from build123d import *

# Parameters (mm, degrees)
SKETCH_1_R          = 10
EXTRUDE_1_DEPTH     = 65
CUT_EXTRUDE_1_DEPTH = 2.5
SKETCH_3_R          = 17.5
EXTRUDE_2_DEPTH     = 28
SKETCH_4_R          = 1.4
CUT_EXTRUDE_2_DEPTH = 3
SKETCH_5_R          = 1.5
CUT_EXTRUDE_3_DEPTH = 3


with BuildPart() as part:
    # 草图1 → 凸台-拉伸1 (new body)
    with BuildSketch(Plane.XY):
        Circle(SKETCH_1_R)
    extrude(amount=EXTRUDE_1_DEPTH)

    # 草图2 → 切除-拉伸1 (cut)
    with BuildSketch(Plane.ZY.offset(10)):
        with BuildLine():
            Line((30.6, 2.55), (37.6, 2.55))
            ThreePointArc((37.6, 2.55), (40.15, 0), (37.6, -2.55))
            Line((37.6, -2.55), (30.6, -2.55))
            ThreePointArc((30.6, -2.55), (28.05, 0), (30.6, 2.55))
        make_face()
    extrude(amount=-CUT_EXTRUDE_1_DEPTH, mode=Mode.SUBTRACT)

    # 草图3 → 凸台-拉伸2 (add)
    with BuildSketch(Plane(origin=(0, 0, 0), x_dir=(-1, 0, 0), z_dir=(0, 0, -1))):
        Circle(SKETCH_3_R)
    extrude(amount=-EXTRUDE_2_DEPTH)

    # 草图4 → 切除-拉伸2 (cut)
    with BuildSketch(Plane.XY.offset(65)):
        with Locations((0, 7)):
            Circle(SKETCH_4_R)
        with Locations((7, 0)):
            Circle(SKETCH_4_R)
        with Locations((0, -7)):
            Circle(SKETCH_4_R)
        with Locations((-7, 0)):
            Circle(SKETCH_4_R)
    extrude(amount=-CUT_EXTRUDE_2_DEPTH, mode=Mode.SUBTRACT)

    # 草图5 → 切除-拉伸3 (cut)
    with BuildSketch(Plane.XY.offset(65)):
        Circle(SKETCH_5_R)
    extrude(amount=-CUT_EXTRUDE_3_DEPTH, mode=Mode.SUBTRACT)


solid = part.part
Input: part model. Units: mm. Frame: model coordinates. A direction names the side the tool comes from. Coordinates: 2 decimals unless noted, no trailing zeros. Order: outer loops, then holes, each group sorted by start corner. A loop starts at its lowest first (then second) coordinate and runs counter-clockwise, first axis right, second up. Notation, with made-up numbers: M 51,58 L 100,58 A8 cw 100,67 Z; hole C 83.25,35.25 d5. An arc over 180 degrees is marked long. Answer as CSV lines item,"result".
1. Section B-B (x = -3). Return the cut outline in (y, z).
Reported:
outline,"M -17.24,0 L 17.24,0 L 17.24,28 L 9.54,28 L 9.54,65 L -9.54,65 L -9.54,28 L -17.24,28 Z"
2. First-contact query: P1, Ø2.5, axis at x = 7, y = 0, coming from the +Z side; P2, Ø1.7, axis at x = -9, z = 35, coming from the -Y side; P3, Ø2, axis at y = 2, z = 15.5, coming from the -X side. Flat tips, straight axial feed; report the tip coordinate or a pass-through.
Reported:
P1,"z = 62"
P2,"y = -5.79"
P3,"x = -17.47"
3. Section D-D (z = 21). Return the cut outline in (x, y).
Reported:
outline,"C 0,0 d35"
4. Material intervals for line 1 (Y direction, x = 0, z = 63.3); line 2 (Z direction, x = 11.5, y = -10.5); line 3 (Y direction, x = -8.5, z = 31.5), sorted ascending. Write a range as from..to.
Reported:
line 1,"-10..-8.4, -5.6..-1.5, 1.5..5.6, 8.4..10"
line 2,"0..28"
line 3,"-5.27..-2.55, 2.55..5.27"
5. Access query for faces 4 (the flat face through (0, 0, 62)), 5 (the flat face through (-7.5, 0, 34)), 6 (the flat face through (0, 0, 0)). Directions: +Z, -Z, +X, -X, +Y, -Y. A direction counts if a zero-diameter tool reaches every point of the face in a straight line with its end or side. Return the directions, or none.
Reported:
face 4,"+Z"
face 5,"-X"
face 6,"-Z, +X, -X, +Y, -Y"
6. Pull-direction query (Y, two-part tool) for faces 1 (the flat face through (0, -2, 65)), 2 (the cylindrical face through (13.887, -10.648, 13.804)), 3 (the cylindrical face through (-8.4, 0.06, 63.52)); classes: released by +Y, released by -Y, zero draft, split by the parting line, or undercut.
Reported:
face 1,"zero draft"
face 2,"split by the parting line"
face 3,"undercut"
7. Section C-C (y = -7). Return the cut outline in (x, z).
Reported:
outline,"M -16.04,0 L 16.04,0 L 16.04,28 L 7.14,28 L 7.14,65 L 1.4,65 L 1.4,62 L -1.4,62 L -1.4,65 L -7.14,65 L -7.14,28 L -16.04,28 Z"
8. Section A-A (z = 60.5). Return the cut outline in (x, y).
Reported:
outline,"C 0,0 d20"
